```python
from build123d import *

# Parameters (mm, degrees)
SKETCH1_W           = 40
SKETCH1_H           = 81.992065469
BOSS_EXTRUDE4_DEPTH = 5
CHAMFER3_SIZE       = 2.5
CHAMFER4_SIZE       = 2.5
CHAMFER5_SIZE       = 2.5
CHAMFER6_SIZE       = 2.5
SKETCH5_R           = 1.5
CUT_EXTRUDE5_DEPTH  = 0.5


with BuildPart() as part:
    # Sketch1 → Boss-Extrude4 (new body)
    with BuildSketch(Plane(origin=(0, 0, 0), x_dir=(1, 0, 0), z_dir=(0, 1, 0))):
        with Locations((20, 40.996032735)):
            Rectangle(SKETCH1_W, SKETCH1_H)
    extrude(amount=BOSS_EXTRUDE4_DEPTH)

    # Chamfer3
    chamfer3_edges = [part.edges().sort_by_distance(p)[0] for p in [
        (40, 2.5, -81.992065469),
    ]]
    chamfer(chamfer3_edges, length=CHAMFER3_SIZE)

    # Chamfer4
    chamfer4_edges = [part.edges().sort_by_distance(p)[0] for p in [
        (0, 2.5, -81.992065469),
    ]]
    chamfer(chamfer4_edges, length=CHAMFER4_SIZE)

    # Chamfer5
    chamfer5_edges = [part.edges().sort_by_distance(p)[0] for p in [
        (0, 2.5, 0),
    ]]
    chamfer(chamfer5_edges, length=CHAMFER5_SIZE)

    # Chamfer6
    chamfer6_edges = [part.edges().sort_by_distance(p)[0] for p in [
        (40, 2.5, 0),
    ]]
    chamfer(chamfer6_edges, length=CHAMFER6_SIZE)

    # Sketch5 → Cut-Extrude5 (cut)
    with BuildSketch(Plane(origin=(0, 0, 0), x_dir=(1, 0, 0), z_dir=(0, 1, 0))):
        with BuildLine():
            Line((7.5, 62.992065469), (32.5, 62.992065469))
            ThreePointArc((32.5, 62.992065469), (39.5, 69.992065469), (32.5, 76.992065469))
            Line((32.5, 76.992065469), (7.5, 76.992065469))
            ThreePointArc((7.5, 76.992065469), (0.5, 69.992065469), (7.5, 62.992065469))
        make_face()
        with Locations(Location((36.469361294, 69.992065469, 0), (0, 0, 270))):
            Circle(SKETCH5_R, mode=Mode.SUBTRACT)
    extrude(amount=CUT_EXTRUDE5_DEPTH, mode=Mode.SUBTRACT)


solid = part.part
```
CAD build for the part. Positions are in the model's coordinates, mm. A direction names the side the tool comes from. Coordinates: 2 decimals unless noted, no trailing zeros. Loops run counter-clockwise (first coordinate to the right, second up) from the corner with the lowest first, then second, coordinate; pieces in that order, holes last. Notation, with made-up numbers: (-23.75, -38) - (20.25, -38) arc R23 ccw to (20.25, -30) - close; hole circle Ø4 at (-32, -13). An arc over 180 degrees is marked (long way). Return JSON: item names as keys, results as strings.
1. Probe L1, parallel to Y at x = 18.5, z = -64. List the from-to ranges inside material, lowest first. Write a range as from..to.
Result:
{"L1": "y = 0.5..5"}
2. Drop a flat-ended pin along its axis: pin 1 (4 mm diameter, centred on x = 28.5, z = -71, fed in from -Y). Give the stop position or say it passes through.
Result:
{"pin 1": "stops at y = 0.5"}
3. Mould opens along Z. For faces 3 (the flat face through (0, 2, -40)), 4 (the flat face through (20, 2, -81.992)), 5 (the cylindrical face through (0.5, 0.2, -70.1)) say: released by +Z, released by -Z, zero draft, split by the parting line, or undercut.
Result:
{"face 3": "zero draft", "face 4": "released by -Z", "face 5": "undercut"}
4. Band-saw the part on A-A (x = 25). Give the cut face in (y, z).
Result:
{"outline": "(0, -81.99) - (5, -81.99) - (5, 0) - (0, 0) - (0, -62.99) - (0.5, -62.99) - (0.5, -76.99) - (0, -76.99) - close"}
5. 3-axis set-ups, long thin cutter, end or side, ignore diameter. For faces 1 (the flat face through (20, 0.5, -70)), 2 (the flat face through (40, 2, -40)): which of +Z, -Z, +X, -X, +Y, -Y reach the whole face in a straight line?
Result:
{"face 1": "-Y", "face 2": "+Z, -Z, +X, +Y, -Y"}
6. Band-saw the part on B-B (z = -65). Give the cut face in (x, y).
Result:
{"outline": "(0, 0) - (2.59, 0) - (2.59, 0.5) - (37.41, 0.5) - (37.41, 0) - (40, 0) - (40, 5) - (0, 5) - close"}
